from build123d import *

# Parameters (mm, degrees)
BOSS_EXTRUDE1_DEPTH = 101.6


with BuildPart() as part:
    # Sketch1 → Boss-Extrude1 (new body)
    with BuildSketch(Plane.XY):
        with BuildLine():
            Line((76.2, 500), (76.2, 609.6))
            Line((76.2, 609.6), (0, 609.6))
            Line((0, 609.6), (0, 0))
            Line((0, 0), (50.8, 0))
            Line((50.8, 0), (50.8, 38.1))
            Line((50.8, 38.1), (139.7, 38.1))
            Line((139.7, 38.1), (139.7, 0))
            Line((139.7, 0), (438.1, 0))
            Line((438.1, 0), (438.1, 38.1))
            Line((438.1, 38.1), (527, 38.1))
            Line((527, 38.1), (527, 0))
            Line((527, 0), (825.4, 0))
            Line((825.4, 0), (825.4, 38.1))
            Line((825.4, 38.1), (914.3, 38.1))
            Line((914.3, 38.1), (914.3, 0))
            Line((914.3, 0), (965.1, 0))
            Line((965.1, 0), (965.1, 609.6))
            Line((965.1, 609.6), (888.9, 609.6))
            Line((888.9, 609.6), (888.9, 500))
            ThreePointArc((888.9, 500), (482.55, 93.65), (76.2, 500))
        make_face()
    extrude(amount=BOSS_EXTRUDE1_DEPTH)


solid = part.part
Could you check a few things on this model? Use its own coordinates, in mm. A direction names the side the tool comes from. Give positions to 0.01 mm unless a question says otherwise; leave off trailing zeros. Order: outer loops, then holes, each group sorted by start corner. A loop starts at its lowest first (then second) coordinate and runs counter-clockwise, first axis right, second up.
1. Suppose I cut it at B-B (z = 64.5). List the corners of the cut face in (x, y) for me.
2. Suppose I cut it at D-D (y = 165.5). List the corners of the cut face in (x, z) for me, plus the area to 3 significant figures.
3. Will these pins go through, and if not, where does the flat tip stop? P1, Ø12, axis at x = 688, z = 44, coming from the +Y side; P2, Ø10, axis at x = 452.5, z = 89, coming from the -Y side.
4. Suppose I cut it at A-A (y = 320.5). List the corners of the cut face in (x, z) for me.
5. I need wall thicknesses on L1, parallel to X at y = 559.5, z = 27; L2, parallel to Y at x = 69, z = 91.5; L3, parallel to X at y = 163.5, z = 67.5. Which ranges of each line are inside material? Lowest first, please.
6. For faces 1 (the flat face through (674, 0, 50)), 2 (the flat face through (76.2, 554, 50)), 3 (the flat face through (482, 38.1, 50)), which set-ups out of +Z, -Z, +X, -X, +Y, -Y let a thin tool reach every point of the face, with its end or its side?
7. We'd pull the mould along X, two halves only. Please class faces 4 (the flat face through (583, 106, 0)), 5 (the flat face through (888.9, 556, 50)), 6 (the flat face through (50.8, 19, 50)), 7 (the flat face through (0, 309, 50)): pulls with the +X half, pulls with the -X half, needs draft (parallel to the pull), parting line crosses it, or undercut.
8. Suppose I cut it at C-C (x = 482.55). List the corners of the cut face in (y, z) for me, plus the area to 3 significant figures.
Solved:
1. outline: (0, 0) - (50.8, 0) - (50.8, 38.1) - (139.7, 38.1) - (139.7, 0) - (438.1, 0) - (438.1, 38.1) - (527, 38.1) - (527, 0) - (825.4, 0) - (825.4, 38.1) - (914.3, 38.1) - (914.3, 0) - (965.1, 0) - (965.1, 609.6) - (888.9, 609.6) - (888.9, 500) arc R406.35 cw to (76.2, 500) - (76.2, 609.6) - (0, 609.6) - close
2. outline: (0, 0) - (251.83, 0) - (251.83, 101.6) - (0, 101.6) - close; (713.27, 0) - (965.1, 0) - (965.1, 101.6) - (713.27, 101.6) - close
2. area: 51,200 mm2
3. P1: stops at y = 153
3. P2: stops at y = 38.1
4. outline: (0, 0) - (118, 0) - (118, 101.6) - (0, 101.6) - close; (847.1, 0) - (965.1, 0) - (965.1, 101.6) - (847.1, 101.6) - close
5. L1: x = 0 to 76.2, 888.9 to 965.1
5. L2: y = 38.1 to 609.6
5. L3: x = 0 to 254.76, 710.34 to 965.1
6. face 1: +Z, -Z, +X, -X, -Y
6. face 2: +Z, -Z, +Y
6. face 3: +Z, -Z, -Y
7. face 4: needs draft
7. face 5: undercut
7. face 6: undercut
7. face 7: pulls with the -X half
8. outline: (38.1, 0) - (93.65, 0) - (93.65, 101.6) - (38.1, 101.6) - close
8. area: 5,640 mm2
